```python
from build123d import *

# Parameters (mm, degrees)
SALIENTE_EXTRUIR1_DEPTH = 6
CORTAR_EXTRUIR1_DEPTH   = 2
CORTAR_EXTRUIR3_START   = -6
CORTAR_EXTRUIR3_DEPTH   = 2
CROQUIS5_R              = 1.5
CORTAR_EXTRUIR4_DEPTH   = 32
CORTAR_EXTRUIR5_DEPTH   = 2
CORTAR_EXTRUIR7_DEPTH   = 2
CROQUIS9_R              = 1.5
CORTAR_EXTRUIR8_DEPTH   = 2
CORTAR_EXTRUIR9_DEPTH   = 2
CORTAR_EXTRUIR10_DEPTH  = 2
CROQUIS12_R             = 1.5
CORTAR_EXTRUIR11_DEPTH  = 2
CROQUIS13_R             = 4.1
CORTAR_EXTRUIR12_DEPTH  = 4
CROQUIS14_R             = 1.5
CORTAR_EXTRUIR13_DEPTH  = 4
CROQUIS15_R             = 1.5
CROQUIS15_R_2           = 4
CORTAR_EXTRUIR14_DEPTH  = 4
CROQUIS16_R             = 1.5
CORTAR_EXTRUIR15_DEPTH  = 4
CROQUIS17_W             = 10
CROQUIS17_H             = 25
CORTAR_EXTRUIR16_DEPTH  = 11.3
CROQUIS18_R             = 1.5
CORTAR_EXTRUIR17_DEPTH  = 14


with BuildPart() as part:
    # Croquis1 → Saliente-Extruir1 (new body)
    with BuildSketch(Plane(origin=(0, 0, 0), x_dir=(1, 0, 0), z_dir=(0, 1, 0))):
        Polygon((0, 0), (174, 0), (174, 20), (154, 20), (154, 85), (174, 85), (174, 160), (154, 160), (154, 130), (20, 130), (20, 160), (0, 160), (0, 85), (20, 85), (20, 20), (0, 20), align=None)
    extrude(amount=SALIENTE_EXTRUIR1_DEPTH)

    # Croquis3 → Cortar-Extruir1 (cut)
    with BuildSketch(Plane(origin=(0, 6, 0), x_dir=(1, 0, 0), z_dir=(0, 1, 0))):
        Polygon((13.1, 141.25), (11.55, 143.934678752), (8.45, 143.934678752), (6.9, 141.25), (8.45, 138.565321248), (11.55, 138.565321248), align=None)
        Polygon((13.1, 103.75), (11.55, 106.434678752), (8.45, 106.434678752), (6.9, 103.75), (8.45, 101.065321248), (11.55, 101.065321248), align=None)
        Polygon((13.1, 10), (11.55, 12.684678752), (8.45, 12.684678752), (6.9, 10), (8.45, 7.315321248), (11.55, 7.315321248), align=None)
        Polygon((162.45, 101.065321248), (160.9, 103.75), (162.45, 106.434678752), (165.55, 106.434678752), (167.1, 103.75), (165.55, 101.065321248), align=None)
        Polygon((162.45, 138.565321248), (160.9, 141.25), (162.45, 143.934678752), (165.55, 143.934678752), (167.1, 141.25), (165.55, 138.565321248), align=None)
        Polygon((162.45, 7.315321248), (160.9, 10), (162.45, 12.684678752), (165.55, 12.684678752), (167.1, 10), (165.55, 7.315321248), align=None)
    extrude(amount=-CORTAR_EXTRUIR1_DEPTH, mode=Mode.SUBTRACT)

    # Croquis4 → Cortar-Extruir3 (cut)
    with BuildSketch(Plane(origin=(0, 6, 0), x_dir=(1, 0, 0), z_dir=(0, 1, 0)).offset(CORTAR_EXTRUIR3_START)):
        Polygon((6.9, 10), (8.45, 7.315321248), (11.55, 7.315321248), (13.1, 10), (11.55, 12.684678752), (8.45, 12.684678752), align=None)
        Polygon((6.9, 103.75), (8.45, 101.065321248), (11.55, 101.065321248), (13.1, 103.75), (11.55, 106.434678752), (8.45, 106.434678752), align=None)
        Polygon((6.9, 141.25), (8.45, 138.565321248), (11.55, 138.565321248), (13.1, 141.25), (11.55, 143.934678752), (8.45, 143.934678752), align=None)
        Polygon((162.45, 143.934678752), (160.9, 141.25), (162.45, 138.565321248), (165.55, 138.565321248), (167.1, 141.25), (165.55, 143.934678752), align=None)
        Polygon((162.45, 106.434678752), (160.9, 103.75), (162.45, 101.065321248), (165.55, 101.065321248), (167.1, 103.75), (165.55, 106.434678752), align=None)
        Polygon((162.45, 12.684678752), (160.9, 10), (162.45, 7.315321248), (165.55, 7.315321248), (167.1, 10), (165.55, 12.684678752), align=None)
    extrude(amount=CORTAR_EXTRUIR3_DEPTH, mode=Mode.SUBTRACT)

    # Croquis5 → Cortar-Extruir4 (cut)
    with BuildSketch(Plane(origin=(0, 6, 0), x_dir=(1, 0, 0), z_dir=(0, 1, 0))):
        with Locations(Location((10, 141.25, 0), (0, 0, 270))):
            Circle(CROQUIS5_R)
        with Locations(Location((10, 103.75, 0), (0, 0, 270))):
            Circle(CROQUIS5_R)
        with Locations(Location((10, 10, 0), (0, 0, 270))):
            Circle(CROQUIS5_R)
        with Locations(Location((164, 103.75, 0), (0, 0, 270))):
            Circle(CROQUIS5_R)
        with Locations(Location((164, 141.25, 0), (0, 0, 270))):
            Circle(CROQUIS5_R)
        with Locations(Location((164, 10, 0), (0, 0, 270))):
            Circle(CROQUIS5_R)
    extrude(amount=-CORTAR_EXTRUIR4_DEPTH, mode=Mode.SUBTRACT)

    # Croquis6 → Cortar-Extruir5 (cut)
    with BuildSketch(Plane(origin=(0, 6, 0), x_dir=(1, 0, 0), z_dir=(0, 1, 0))):
        Polygon((53.15, 10), (51.6, 12.684678752), (48.5, 12.684678752), (46.95, 10), (48.5, 7.315321248), (51.6, 7.315321248), align=None)
        Polygon((127.05, 10), (125.5, 12.684678752), (122.4, 12.684678752), (120.85, 10), (122.4, 7.315321248), (125.5, 7.315321248), align=None)
    extrude(amount=-CORTAR_EXTRUIR5_DEPTH, mode=Mode.SUBTRACT)

    # Croquis7 → Cortar-Extruir7 (cut)
    with BuildSketch(Plane.XZ):
        Polygon((53.15, -10), (51.6, -7.315321248), (48.5, -7.315321248), (46.95, -10), (48.5, -12.684678752), (51.6, -12.684678752), align=None)
        Polygon((127.05, -10), (125.5, -7.315321248), (122.4, -7.315321248), (120.85, -10), (122.4, -12.684678752), (125.5, -12.684678752), align=None)
    extrude(amount=-CORTAR_EXTRUIR7_DEPTH, mode=Mode.SUBTRACT)

    # Croquis9 → Cortar-Extruir8 (cut)
    with BuildSketch(Plane.XZ.offset(-2)):
        with Locations(Location((123.95, -10, 0), (0, 0, 270))):
            Circle(CROQUIS9_R)
        with Locations(Location((50.05, -10, 0), (0, 0, 270))):
            Circle(CROQUIS9_R)
    extrude(amount=-CORTAR_EXTRUIR8_DEPTH, mode=Mode.SUBTRACT)

    # Croquis10 → Cortar-Extruir9 (cut)
    with BuildSketch(Plane(origin=(0, 6, 0), x_dir=(1, 0, 0), z_dir=(0, 1, 0))):
        Polygon((33.1, 66.25), (31.55, 68.934678752), (28.45, 68.934678752), (26.9, 66.25), (28.45, 63.565321248), (31.55, 63.565321248), align=None)
        Polygon((147.1, 66.25), (145.55, 68.934678752), (142.45, 68.934678752), (140.9, 66.25), (142.45, 63.565321248), (145.55, 63.565321248), align=None)
    extrude(amount=-CORTAR_EXTRUIR9_DEPTH, mode=Mode.SUBTRACT)

    # Croquis11 → Cortar-Extruir10 (cut)
    with BuildSketch(Plane.XZ):
        Polygon((145.55, -63.565321248), (147.1, -66.25), (145.55, -68.934678752), (142.45, -68.934678752), (140.9, -66.25), (142.45, -63.565321248), align=None)
        Polygon((31.55, -63.565321248), (33.1, -66.25), (31.55, -68.934678752), (28.45, -68.934678752), (26.9, -66.25), (28.45, -63.565321248), align=None)
    extrude(amount=-CORTAR_EXTRUIR10_DEPTH, mode=Mode.SUBTRACT)

    # Croquis12 → Cortar-Extruir11 (cut)
    with BuildSketch(Plane.XZ.offset(-2)):
        with Locations(Location((144, -66.25, 0), (0, 0, 270))):
            Circle(CROQUIS12_R)
        with Locations(Location((30, -66.25, 0), (0, 0, 270))):
            Circle(CROQUIS12_R)
    extrude(amount=-CORTAR_EXTRUIR11_DEPTH, mode=Mode.SUBTRACT)

    # Croquis13 → Cortar-Extruir12 (cut)
    with BuildSketch(Plane(origin=(0, 6, 0), x_dir=(1, 0, 0), z_dir=(0, 1, 0))):
        with Locations(Location((117.01, 105, 0), (0, 0, 270))):
            Circle(CROQUIS13_R)
        with Locations(Location((56.99, 105, 0), (0, 0, 90))):
            Circle(CROQUIS13_R)
    extrude(amount=-CORTAR_EXTRUIR12_DEPTH, mode=Mode.SUBTRACT)

    # Croquis14 → Cortar-Extruir13 (cut)
    with BuildSketch(Plane(origin=(0, 2, 0), x_dir=(1, 0, 0), z_dir=(0, 1, 0))):
        with Locations(Location((117.01, 105, 0), (0, 0, 270))):
            Circle(CROQUIS14_R)
        with Locations(Location((56.99, 105, 0), (0, 0, 270))):
            Circle(CROQUIS14_R)
    extrude(amount=-CORTAR_EXTRUIR13_DEPTH, mode=Mode.SUBTRACT)

    # Croquis15 → Cortar-Extruir14 (cut)
    with BuildSketch(Plane(origin=(0, 6, 0), x_dir=(1, 0, 0), z_dir=(0, 1, 0))):
        with Locations(Location((56.99, 105, 0), (0, 0, 270))):
            Circle(CROQUIS15_R)
        with Locations(Location((56.99, 73.98, 0), (0, 0, 270))):
            Circle(CROQUIS15_R_2)
        with Locations(Location((117.01, 105, 0), (0, 0, 270))):
            Circle(CROQUIS15_R)
        with Locations(Location((117.01, 73.98, 0), (0, 0, 270))):
            Circle(CROQUIS15_R_2)
    extrude(amount=-CORTAR_EXTRUIR14_DEPTH, mode=Mode.SUBTRACT)

    # Croquis16 → Cortar-Extruir15 (cut)
    with BuildSketch(Plane(origin=(0, 2, 0), x_dir=(1, 0, 0), z_dir=(0, 1, 0))):
        with Locations(Location((56.99, 73.98, 0), (0, 0, 270))):
            Circle(CROQUIS16_R)
        with Locations(Location((117.01, 73.98, 0), (0, 0, 270))):
            Circle(CROQUIS16_R)
    extrude(amount=-CORTAR_EXTRUIR15_DEPTH, mode=Mode.SUBTRACT)

    # Croquis17 → Cortar-Extruir16 (cut)
    with BuildSketch(Plane(origin=(0, 6, 0), x_dir=(1, 0, 0), z_dir=(0, 1, 0))):
        with Locations((35, 97.543907688)):
            Rectangle(CROQUIS17_W, CROQUIS17_H)
        with Locations((139, 97.543907688)):
            Rectangle(CROQUIS17_W, CROQUIS17_H)
    extrude(amount=-CORTAR_EXTRUIR16_DEPTH, mode=Mode.SUBTRACT)

    # Croquis18 → Cortar-Extruir17 (cut)
    with BuildSketch(Plane(origin=(0, 6, 0), x_dir=(1, 0, 0), z_dir=(0, 1, 0))):
        with Locations(Location((38, 122, 0), (0, 0, 270))):
            Circle(CROQUIS18_R)
        with Locations(Location((62, 122, 0), (0, 0, 270))):
            Circle(CROQUIS18_R)
    extrude(amount=-CORTAR_EXTRUIR17_DEPTH, mode=Mode.SUBTRACT)


solid = part.part
```
Model file for the job. Use its own axes, mm. A direction names the side the tool comes from. Give positions to 0.01 mm unless a question says otherwise; leave off trailing zeros. Write each loop counter-clockwise with the first axis right and the second up, starting at its lowest first coordinate (ties: lowest second). Pieces come first, ordered by that corner, then holes. Notation, with made-up numbers: (65.25, 89) -> (87.25, 89) arc R21 cw to (87.25, 102) -> close; hole circle Ø3 at (73.5, 13.5). An arc over 180 degrees is marked (long way). Use CSV: the item, a comma, the result in double quotes. Start each with the question number.
1) Cut at A-A on z = -91.5. List the corners of the cut face in (x, y), plus the area to 3 significant figures.
2) Two-plate mould, pull along X, no slides. Class faces 4 (the flat face through (165.3, 2, -102.6)), 5 (the flat face through (164, 3, -20)), 6 (the flat face through (174, 3, -122)): released by +X, released by -X, zero draft, split by the parting line, or undercut.
3) Cut at C-C on z = -38. List the corners of the cut face in (x, y).
4) Drill centre lines: L1, parallel to X at y = 4.35, z = -122; L2, parallel to X at y = 0.35, z = -92; L3, parallel to Z at x = 161, y = 0.65. Where is each one in solid material? Low to high.
5) Tool access for faces 1 (the flat face through (165.3, 2, -8.8)), 2 (the flat face through (31.3, 4, -67.5)), 3 (the flat face through (10, 3, -20)): list every direction of +Z, -Z, +X, -X, +Y, -Y with a clear straight run to the whole face (end or side of a thin tool).
6) Cut at B-B on x = 84.5. List the corners of the cut face in (y, z), plus the area to 3 significant figures.
7) Pin check, flat tips, straight feed: P1, Ø1.6, axis at x = 50, y = 5, coming from the -Z side; P2, Ø2, axis at y = 4, z = -36, coming from the -X side; P3, Ø2.5, axis at x = 117.01, z = -105, coming from the +Y side. Stop position of each tip, or through.
Final values:
1,outline,"(0, 0) -> (30, 0) -> (30, 6) -> (0, 6) -> close; (40, 0) -> (134, 0) -> (134, 6) -> (40, 6) -> close; (144, 0) -> (174, 0) -> (174, 6) -> (144, 6) -> close"
1,area,"924 mm2"
2,face 4,"undercut"
2,face 5,"zero draft"
2,face 6,"released by +X"
3,outline,"(20, 0) -> (154, 0) -> (154, 6) -> (20, 6) -> close"
4,L1,"x = 0 to 36.5, 39.5 to 60.5, 63.5 to 174"
4,L2,"x = 0 to 30, 40 to 134, 144 to 174"
4,L3,"z = -160 to -141.42, -141.08 to -103.92, -103.58 to -85, -20 to -10.17, -9.83 to 0"
5,face 1,"-Y"
5,face 2,"+Y"
5,face 3,"-X, +Y, -Y"
6,outline,"(0, -130) -> (6, -130) -> (6, 0) -> (0, 0) -> close"
6,area,"780 mm2"
7,P1,"stops at z = -130"
7,P2,"stops at x = 20"
7,P3,"passes through"
